Can you work these out from the model? Positions are in its coordinate system, mm. A direction names the side the tool comes from. Round coordinates to 2 decimals unless told otherwise and drop trailing zeros. Write each loop counter-clockwise with the first axis right and the second up, starting at its lowest first coordinate (ties: lowest second). Pieces come first, ordered by that corner, then holes.
Q1. If we section it at A-A (z = 0): Please give me the cut outline in (x, y) (3 decimals), plus the area to 3 significant figures.
Q2. For faces 1 (the cylindrical face through (10.396, 5.014, 7.501)), 2 (the cylindrical face through (6.1, 4, -10.4)), 3 (the flat face through (-6.55, 8, 0)), 4 (the cylindrical face through (-8.9, 4.7, -10.5)), which set-ups out of +Z, -Z, +X, -X, +Y, -Y let a thin tool reach every point of the face, with its end or its side?
Q3. Please list where these lines run through material, in increasing order: line 1 along Y through (x, z) = (0, -10.25) (3 decimals); line 2 along Z through (x, y) = (2, 6.75).
Q4. If we section it at D-D (x = -9.25): Please give me the cut outline in (y, z) (3 decimals), plus the area to 3 significant figures.
Q5. We'd pull the mould along Z, two halves only. Please class faces 5 (the flat face through (0, 7, 12.9)), 6 (the cylindrical face through (-6.1, 4, 10.4)), 7 (the cylindrical face through (10.396, 5.014, -7.501)), 8 (the cylindrical face through (-8.517, 2.665, -0.446)): +Z half, -Z half, draft (parallel to the pull), parting line (faces both ways), or undercut.
Q6. If we section it at C-C (y = 6): Give the number of separate pieces and of enclosed holes in the cut face, plus the area to 3 significant figures.
Q7. If we section it at B-B (z = -9.25): Please give me the cut outline in (x, y) (3 decimals), plus the area to 3 significant figures.
Q8. I'm going to push flat-ended pins straight in: pin 1 Ø1.5 at (x, y) = (1, 3) entering from +Z; pin 2 Ø1.4 at (x, y) = (6.68, 4.67) entering from +Z; pin 3 Ø1.5 at (x, z) = (-1.5, -4) entering from +Y; pin 4 Ø2 at (x, z) = (9.725, 9.725) entering from +Y. Where does each tip first touch, or does it pass through?
from build123d import *

# Parameters (mm, degrees)
SKETCH1_W             = 25.8
SKETCH1_H             = 25.8
BOSS_EXTRUDE1_DEPTH   = 9.525
SKETCH3_R             = 2.0574
CUT_EXTRUDE3_DEPTH    = 8.89
SKETCH7_R             = 2.0574
CUT_EXTRUDE5_DEPTH    = 8.89
CUT_EXTRUDE10_DEPTH   = 3.9376
CUT_EXTRUDE11_DEPTH   = 0.28
F_4_40_TAPPED_HOLE2_D = 2.2606
CUT_EXTRUDE12_DEPTH   = 2.032


with BuildPart() as part:
    # Sketch1 → Boss-Extrude1 (new body)
    with BuildSketch(Plane(origin=(0, 0, 0), x_dir=(1, 0, 0), z_dir=(0, 1, 0))):
        Rectangle(SKETCH1_W, SKETCH1_H)
    extrude(amount=BOSS_EXTRUDE1_DEPTH)

    # Sketch3 → Cut-Extrude3 (cut)
    with BuildSketch(Plane.ZY.offset(12.9)):
        with Locations((0, 4.6736)):
            Circle(SKETCH3_R)
    cut_extrude3 = extrude(amount=-CUT_EXTRUDE3_DEPTH, mode=Mode.SUBTRACT)

    # Mirror1: Cut-Extrude3 across plane
    add(cut_extrude3.mirror(Plane(origin=(0, 0, 0), x_dir=(0, 0, 1), z_dir=(1, 0, 0))), mode=Mode.SUBTRACT)

    # Sketch7 → Cut-Extrude5 (cut)
    with BuildSketch(Plane(origin=(0, 0, -12.9), x_dir=(-1, 0, 0), z_dir=(0, 0, -1))):
        with Locations((0, 4.6736)):
            Circle(SKETCH7_R)
    cut_extrude5 = extrude(amount=-CUT_EXTRUDE5_DEPTH, mode=Mode.SUBTRACT)

    # Mirror2: Cut-Extrude5 across plane
    add(cut_extrude5.mirror(Plane.XY), mode=Mode.SUBTRACT)

    # Sketch14 → Cut-Extrude10 (cut)
    with BuildSketch(Plane(origin=(0, 9.525, 0), x_dir=(1, 0, 0), z_dir=(0, 1, 0))):
        with BuildLine():
            Line((-5.75625, -6.55), (5.75625, -6.55))
            ThreePointArc((5.75625, -6.55), (6.317516008, -6.317516008), (6.55, -5.75625))
            Line((6.55, -5.75625), (6.55, 5.75625))
            ThreePointArc((6.55, 5.75625), (6.317516008, 6.317516008), (5.75625, 6.55))
            Line((5.75625, 6.55), (-5.75625, 6.55))
            ThreePointArc((-5.75625, 6.55), (-6.317516008, 6.317516008), (-6.55, 5.75625))
            Line((-6.55, 5.75625), (-6.55, -5.75625))
            ThreePointArc((-6.55, -5.75625), (-6.317516008, -6.317516008), (-5.75625, -6.55))
        make_face()
    extrude(amount=-CUT_EXTRUDE10_DEPTH, mode=Mode.SUBTRACT)

    # Sketch15 → Cut-Extrude11 (cut)
    with BuildSketch(Plane(origin=(0, 5.5874, 0), x_dir=(1, 0, 0), z_dir=(0, 1, 0))):
        with BuildLine():
            Line((-2.887467985, 4.01), (2.887467985, 4.01))
            ThreePointArc((2.887467985, 4.01), (4.01, 4.01), (4.01, 2.887467985))
            Line((4.01, 2.887467985), (4.01, -2.887467985))
            ThreePointArc((4.01, -2.887467985), (4.01, -4.01), (2.887467985, -4.01))
            Line((2.887467985, -4.01), (-2.887467985, -4.01))
            ThreePointArc((-2.887467985, -4.01), (-4.01, -4.01), (-4.01, -2.887467985))
            Line((-4.01, -2.887467985), (-4.01, 2.887467985))
            ThreePointArc((-4.01, 2.887467985), (-4.01, 4.01), (-2.887467985, 4.01))
        make_face()
    extrude(amount=-CUT_EXTRUDE11_DEPTH, mode=Mode.SUBTRACT)

    # #4-40 Tapped Hole2 (through all)
    with Locations(Plane(origin=(0, 9.525, 0), x_dir=(1, 0, 0), z_dir=(0, 1, 0))):
        with Locations((9.725, -9.725), (-9.725, -9.725), (-9.725, 9.725), (9.725, 9.725)):
            Hole(F_4_40_TAPPED_HOLE2_D / 2)

    # Sketch22 → #2-56 Tapped Hole1 (revolve, cut)
    with BuildSketch(Plane(origin=(-6.6802, 4.6736, -12.9), x_dir=(0, 1, 0), z_dir=(1, 0, 0))):
        Polygon((0, 0), (0, 5.61416509), (0.889, 5.08), (0.889, 0), align=None)
    f_2_56_tapped_hole1 = revolve(axis=Axis((-6.6802, 4.6736, -19.25), (0, 0, 1)), mode=Mode.SUBTRACT)

    # Mirror7: #2-56 Tapped Hole1 across plane
    add(f_2_56_tapped_hole1.mirror(Plane(origin=(0, 0, 0), x_dir=(0, 0, 1), z_dir=(1, 0, 0))), mode=Mode.SUBTRACT)

    # Mirror8: #2-56 Tapped Hole1 across plane
    add(f_2_56_tapped_hole1.mirror(Plane.XY), mode=Mode.SUBTRACT)

    # Mirror8 copy 1 sketch → Mirror8 copy 1 (revolve, cut)
    with BuildSketch(Plane(origin=(6.6802, 4.6736, 12.9), x_dir=(0, 1, 0), z_dir=(-1, 0, 0))):
        Polygon((0, 0), (0, 5.61416509), (0.889, 5.08), (0.889, 0), align=None)
    revolve(axis=Axis((6.6802, 4.6736, 19.25), (0, 0, -1)), mode=Mode.SUBTRACT)

    # Sketch24 → #2-56 Tapped Hole2 (revolve, cut)
    with BuildSketch(Plane(origin=(12.9, 4.6736, -6.6802), x_dir=(0, 0, -1), z_dir=(0, 1, 0))):
        Polygon((0, 0), (0, 5.61416509), (0.889, 5.08), (0.889, 0), align=None)
    f_2_56_tapped_hole2 = revolve(axis=Axis((19.25, 4.6736, -6.6802), (-1, 0, 0)), mode=Mode.SUBTRACT)

    # Mirror9: #2-56 Tapped Hole2 across plane
    add(f_2_56_tapped_hole2.mirror(Plane.XY), mode=Mode.SUBTRACT)

    # Mirror10: #2-56 Tapped Hole2 across plane
    add(f_2_56_tapped_hole2.mirror(Plane(origin=(0, 0, 0), x_dir=(0, 0, 1), z_dir=(1, 0, 0))), mode=Mode.SUBTRACT)

    # Mirror10 copy 1 sketch → Mirror10 copy 1 (revolve, cut)
    with BuildSketch(Plane(origin=(-12.9, 4.6736, 6.6802), x_dir=(0, 0, 1), z_dir=(0, 1, 0))):
        Polygon((0, 0), (0, 5.61416509), (0.889, 5.08), (0.889, 0), align=None)
    revolve(axis=Axis((-19.25, 4.6736, 6.6802), (1, 0, 0)), mode=Mode.SUBTRACT)

    # Sketch25 → Cut-Extrude12 (cut)
    with BuildSketch(Plane(origin=(0, 9.525, 0), x_dir=(1, 0, 0), z_dir=(0, 1, 0))):
        with BuildLine():
            Line((-5.427467966, -6.549999981), (5.427467966, -6.549999981))
            ThreePointArc((5.427467966, -6.549999981), (5.988733973, -6.782483973), (6.549999981, -6.549999981))
            ThreePointArc((6.549999981, -6.549999981), (6.782483973, -5.988733973), (6.549999981, -5.427467966))
            Line((6.549999981, -5.427467966), (6.549999981, 5.427467966))
            ThreePointArc((6.549999981, 5.427467966), (6.782483973, 5.988733973), (6.549999981, 6.549999981))
            ThreePointArc((6.549999981, 6.549999981), (5.988733973, 6.782483973), (5.427467966, 6.549999981))
            Line((5.427467966, 6.549999981), (-5.427467966, 6.549999981))
            ThreePointArc((-5.427467966, 6.549999981), (-5.988733973, 6.782483973), (-6.549999981, 6.549999981))
            ThreePointArc((-6.549999981, 6.549999981), (-6.782483973, 5.988733973), (-6.549999981, 5.427467966))
            Line((-6.549999981, 5.427467966), (-6.549999981, -5.427467966))
            ThreePointArc((-6.549999981, -5.427467966), (-6.782483973, -5.988733973), (-6.549999981, -6.549999981))
            ThreePointArc((-6.549999981, -6.549999981), (-5.988733973, -6.782483973), (-5.427467966, -6.549999981))
        make_face()
    extrude(amount=-CUT_EXTRUDE12_DEPTH, mode=Mode.SUBTRACT)


solid = part.part
A:
1. outline: (-12.9, 0) - (12.9, 0) - (12.9, 2.616) - (4.01, 2.616) - (4.01, 5.307) - (-4.01, 5.307) - (-4.01, 2.616) - (-12.9, 2.616) - close; (-12.9, 6.731) - (-6.55, 6.731) - (-6.55, 9.525) - (-12.9, 9.525) - close; (6.55, 6.731) - (12.9, 6.731) - (12.9, 9.525) - (6.55, 9.525) - close
1. area: 125 mm2
2. face 1: +X
2. face 2: -Z
2. face 3: +Y
2. face 4: +Y, -Y
3. line 1: y = 0 to 2.616, 6.731 to 9.525
3. line 2: z = -12.9 to -6.55, 6.55 to 12.9
4. outline: (0, -12.9) - (9.525, -12.9) - (9.525, -10.751) - (0, -10.751) - close; (0, -8.699) - (9.525, -8.699) - (9.525, 8.699) - (0, 8.699) - close; (0, 10.751) - (9.525, 10.751) - (9.525, 12.9) - (0, 12.9) - close; hole circle Ø4.115 at (4.674, 0); hole circle Ø1.778 at (4.674, -6.68); hole circle Ø1.778 at (4.674, 6.68)
4. area: 188 mm2
5. face 5: +Z half
5. face 6: draft
5. face 7: undercut
5. face 8: undercut
6. separate pieces: 4
6. enclosed holes: 4
6. area: 399 mm2
7. outline: (-12.9, 0) - (-10.751, 0) - (-10.751, 9.525) - (-12.9, 9.525) - close; (-8.699, 0) - (8.699, 0) - (8.699, 9.525) - (-8.699, 9.525) - close; (10.751, 0) - (12.9, 0) - (12.9, 9.525) - (10.751, 9.525) - close; hole circle Ø1.778 at (-6.68, 4.674); hole circle Ø4.115 at (0, 4.674); hole circle Ø1.778 at (6.68, 4.674)
7. area: 188 mm2
8. pin 1: stops at z = 12.9
8. pin 2: stops at z = 7.71
8. pin 3: stops at y = 5.59
8. pin 4: passes through
